Build history of the part. All positions in model axes, mm. A direction names the side the tool comes from. Round coordinates to 2 decimals unless told otherwise and drop trailing zeros. Write each loop counter-clockwise with the first axis right and the second up, starting at its lowest first coordinate (ties: lowest second). Pieces come first, ordered by that corner, then holes.
Item 1: Drop flat-ended pins along their axis: pin 1 Ø0.6 at (x, z) = (-5.5, -0.5) entering from +Y; pin 2 Ø1.5 at (y, z) = (0, 8.5) entering from -X; pin 3 Ø2 at (y, z) = (-3, 5.5) entering from +X. Give the stop position or say it passes through.
Item 2: 3-axis set-ups, long thin cutter, end or side, ignore diameter. For faces 1 (the flat face through (2, -5, 3)), 2 (the flat face through (-6, 2, 1)): which of +Z, -Z, +X, -X, +Y, -Y reach the whole face in a straight line?
Item 3: Wall check: probe 1 along X at (y, z) = (3.25, 0); probe 2 along Z at (x, y) = (0, 1); probe 3 along X at (y, z) = (-2.5, 0). Give the ranges that are in metal, low to high.
Item 4: Band-saw the part on A-A, the plane x = 0. Write the cut outline in (y, z), then the cut area to 3 significant figures.
Item 5: Band-saw the part on D-D, the plane y = 0.5. Write the cut outline in (x, z).
Item 6: Band-saw the part on C-C, the plane z = 1.5. Write the cut outline in (x, y).
Item 7: Band-saw the part on B-B, the plane y = -4. Write the cut outline in (x, z), then the cut area to 3 significant figures.
Autodesk Fusion 360 part; units mm, degrees
sketch "Sketch1" plane through (0, 0, 0) normal (0, 1, 0) x (1, 0, 0)
  circle A0 centre (0, 0) radius 3
  circle A1 centre (0, 0) radius 5
  line L0 (5, -1) -> (7, -1)
  line L1 (7, -1) -> (7, 51)
  line L2 (7, 51) -> (5, 51)
  line L3 (5, 51) -> (5, -1)
  line L4 (5, 25) -> (0, 25) construction
  line L5 (0, 25) -> (0, 0) construction
  line L6 (0, 0) -> (0, -10) construction
  line L7 (0, 5) -> (10, 5) construction
  line L8 (10, 5) -> (10, 0)
  arc A2 (0, -10) -> (10, 0) centre (0, 0) ccw
  line L9 (10, 5) -> (7, 5)
  line L10 (5, 5) -> (0, 5)
  line L11 (-5, 5) -> (0, 5)
  line L12 (-5, 51) -> (-5, -1)
  line L13 (-5, -1) -> (-7, -1)
  line L14 (-7, -1) -> (-7, 51)
  line L15 (-10, 5) -> (-7, 5)
  arc A3 (-10, 0) -> (0, -10) centre (0, 0) ccw
  line L16 (-10, 5) -> (-10, 0)
  dimension "d1" = 6
  dimension "d2" = 10
  dimension "d3" = 2
  dimension "d4" = 52
  dimension "d5" = 25
  dimension "d6" = 10
  dimension "d7" = 10
  dimension "d8" = 5
extrude "Extrude1" add sketch "Sketch1" along normal blind 5 contours A1 | A1 L0 L1 L3 L8 A2 L9 L12 L13 L14 L15 A3 L16 | A1 L3 L10 | A1 L11 L12
sketch "Sketch2" plane through (0, 0, 0) normal (0, -1, 0) x (1, 0, 0)
  circle A0 centre (0, 0) radius 3
  line L0 (-5, 1) -> (-5, -5)
  line L1 (-5, -5) -> (5, -5)
  line L2 (5, -5) -> (5, 1)
  line L3 (5, 1) -> (7, 1)
  line L4 (7, 1) -> (7, -5)
  line L5 (7, -5) -> (10, -5)
  line L6 (10, -5) -> (10, 0)
  arc A1 (10, 0) -> (-10, 0) centre (0, 0) ccw
  line L7 (-10, 0) -> (-10, -5)
  line L8 (-10, -5) -> (-7, -5)
  line L9 (-7, -5) -> (-7, 1)
  line L10 (-7, 1) -> (-5, 1)
  line L11 (10, -5) -> (-10, -5)
extrude "Extrude2" add sketch "Sketch2" along normal blind 5
Results:
1. pin 1: stops at y = 0
1. pin 2: stops at x = -6.32
1. pin 3: stops at x = 8.93
2. face 1: +Z, -Z, +X, -X, -Y
2. face 2: -Z, +Y
3. probe 1: x = -10 to -7, -5 to -3, 3 to 5, 7 to 10
3. probe 2: z = -5 to -3, 3 to 10
3. probe 3: x = -10 to -3, 3 to 10
4. outline: (-5, -5) - (5, -5) - (5, -3) - (-5, -3) - close; (-5, 3) - (5, 3) - (5, 10) - (-5, 10) - close
4. area: 90.0 mm2
5. outline: (-10, -5) - (-7, -5) - (-7, 1) - (-5, 1) - (-5, -5) - (5, -5) - (5, 1) - (7, 1) - (7, -5) - (10, -5) - (10, 0) arc R10 ccw to (-10, 0) - close; hole circle Ø6 at (0, 0)
6. outline: (-9.89, -5) - (-2.6, -5) - (-2.6, 5) - (-9.89, 5) - close; (2.6, -5) - (9.89, -5) - (9.89, 5) - (2.6, 5) - close
7. outline: (-10, -5) - (10, -5) - (10, 0) arc R10 ccw to (-10, 0) - close; hole circle Ø6 at (0, 0)
7. area: 229 mm2
